Autodesk Inventor part; units mm, degrees
ref_plane "YZ Plane" through (0, 0, 0) normal (1, 0, 0) x (0, 1, 0)
ref_plane "XZ Plane" through (0, 0, 0) normal (0, 1, 0) x (-1, 0, 0)
ref_plane "XY Plane" through (0, 0, 0) normal (0, 0, 1) x (1, 0, 0)
sketch "Boceto1" plane through (0, 0, 0) normal (0, 1, 0) x (-1, 0, 0)
  line L0 (0, 0) -> (12.5, 0)
  line L1 (12.5, 0) -> (12.5, -5)
  line L2 (0, -5) -> (0, 0)
  circle A0 centre (6.25, -2.5) radius 1
  arc A1 (8.4861, -5) -> (4.0139, -5) centre (6.25, -7) ccw
  line L3 (12.5, -5) -> (8.4861, -5)
  line L4 (4.0139, -5) -> (0, -5)
  dimension "d1" = 5
  dimension "d2" = 2
  dimension "d4" = 6
extrude "Extrusión1" add sketch "Boceto1" along normal blind 5
sketch "Boceto2" plane through (0, 5, 0) normal (0, 1, 0) x (1, 0, 0)
  line L0 (0, 5) -> (-4.0139, 5)
  arc A0 (-8.4861, 5) -> (-4.0139, 5) centre (-6.25, 7) ccw
  line L1 (-8.4861, 5) -> (-12.5, 5)
  line L2 (-12.5, 5) -> (-12.5, 0)
  line L3 (-12.5, 0) -> (0, 0)
  line L4 (0, 0) -> (0, 5)
  circle A1 centre (-6.25, 2.5) radius 1
  arc A2 (-12.5, 11.25) -> (0, 11.25) centre (-6.25, 11.25) ccw
  arc A3 (0, 15.25) -> (-12.5, 15.25) centre (-6.25, 15.25) ccw
  line L5 (-12.5, 11.25) -> (-12.5, 15.25)
  line L6 (0, 11.25) -> (0, 15.25)
  line L7 (0, 23.25) -> (-12.5, 23.25)
  line L8 (-12.5, 23.25) -> (-12.5, 28.25)
  line L9 (-12.5, 28.25) -> (0, 28.25)
  line L10 (0, 28.25) -> (0, 23.25)
  circle A4 centre (-6.25, 25.75) radius 1
  circle A5 centre (-6.25, 7) radius 27
  circle A6 centre (-6.25, 7) radius 30
  dimension "d8" = 12.5
  dimension "d10" = 12.5
  dimension "d12" = 12.5
  dimension "d13" = 5
  dimension "d14" = 2
  dimension "d15" = 54
  dimension "d17" = 3
extrude "Extrusión2" add sketch "Boceto2" along normal blind 3 contours A5
extrude "Extrusión3" add sketch "Boceto2" against normal blind 5 contours L7 L8 L9 L10
extrude "Extrusión4" add sketch "Boceto2" along normal blind 6.8 contours A6
sketch "Boceto3" plane through (0, 5, 0) normal (0, 1, 0) x (1, 0, 0)
  line L0 (-4.0139, 5) -> (0, 5)
  line L1 (0, 0) -> (-12.5, 0)
  line L2 (0, 5) -> (-12.5, 5)
  line L3 (-12.5, 5) -> (-12.5, 0)
  line L4 (-12.5, 0) -> (0, 0)
  line L5 (0, 0) -> (0, 5)
  line L6 (-12.5, 28.25) -> (0, 28.25)
  line L7 (0, 23.25) -> (-12.5, 23.25)
  line L8 (0, 28.25) -> (-12.5, 28.25)
  line L9 (-12.5, 28.25) -> (-12.5, 23.25)
  line L10 (-12.5, 23.25) -> (0, 23.25)
  line L11 (0, 23.25) -> (0, 28.25)
  circle A0 centre (-6.25, 25.75) radius 1
  circle A1 centre (-6.25, 25.75) radius 1
  circle A2 centre (-6.25, 2.5) radius 1
  circle A3 centre (-6.25, 2.5) radius 1
  dimension "d24" = 12.5
  dimension "d25" = 5
  dimension "d26" = 12.5
  dimension "d27" = 5
  dimension "d28" = 2
  dimension "d29" = 2
extrude "Extrusión5" add sketch "Boceto3" along normal blind 3
sketch "Boceto4" plane through (-6.25, 5, -7) normal (0, -1, 0) x (1, 0, 0)
  circle A0 centre (0, 0) radius 27
  circle A1 centre (0, 0) radius 30
  circle A2 centre (0, 0) radius 27
  point P0 (6.25, 7)
  dimension "d32" = 60
  dimension "d33" = 54
extrude "Extrusión6" add sketch "Boceto4" along normal blind 25
sketch "Boceto5" plane through (-6.25, -20, -7) normal (0, -1, 0) x (1, 0, 0)
  circle A0 centre (0, 0) radius 27
  arc A1 (6.25, -4.25) -> (-6.25, -4.25) centre (0, -4.25) ccw
  line L0 (6.25, -8.25) -> (6.25, -4.25)
  arc A2 (-6.25, -8.25) -> (6.25, -8.25) centre (0, -8.25) ccw
  line L1 (-6.25, -4.25) -> (-6.25, -8.25)
  arc A3 (2.2361, 2) -> (-2.2361, 2) centre (0, 0) ccw
  line L2 (-2.2361, 2) -> (-6.25, 2)
  line L3 (-6.25, 2) -> (-6.25, 7)
  line L4 (-6.25, 7) -> (6.25, 7)
  line L5 (6.25, 7) -> (6.25, 2)
  line L6 (6.25, 2) -> (2.2361, 2)
  line L7 (6.25, -16.25) -> (-6.25, -16.25)
  line L8 (6.25, -21.25) -> (6.25, -16.25)
  line L9 (-6.25, -21.25) -> (6.25, -21.25)
  line L10 (-6.25, -16.25) -> (-6.25, -21.25)
  circle A4 centre (0, 0) radius 30
  circle A5 centre (0, 0) radius 27
  circle A6 centre (0, 0) radius 40
  circle A7 centre (0, 0) radius 30
  line L11 (0, 30) -> (5, 30)
  line L12 (5, 30) -> (-5, 30)
  line L13 (-5, 30) -> (-5, 26.533)
  circle A8 centre (0, 0) radius 27
  line L14 (5, 30) -> (5, 26.533)
  circle A9 centre (0, 0) radius 27
  circle A10 centre (0, 0) radius 30
  dimension "d36" = 80
  dimension "d37" = 5
  dimension "d38" = 10
extrude "Extrusión7" add sketch "Boceto5" along normal blind 3 contours A0 L14 A4 L13 | A0 L13 A4 L14 | A4 L11 L14 | L13 L12 A4 | A6
sketch "Boceto6" plane through (-6.25, -23, -7) normal (0, -1, 0) x (1, 0, 0)
  circle A0 centre (0, 0) radius 30
  circle A1 centre (0, 0) radius 40
  circle A2 centre (0, 0) radius 27
  circle A3 centre (0, 0) radius 30
  circle A4 centre (0, 0) radius 30
  circle A5 centre (0, 0) radius 40
  arc A6 (42.4961, -3.1256) -> (42.4568, 3.1566) centre (40, 0) ccw
  circle A7 centre (40, 0) radius 2.5
  circle A8 centre (0, 0) radius 40
  arc A9 (42.4961, -3.1256) -> (39.2164, -7.8789) centre (48.7365, -10.9396) ccw
  line L0 (39.8, 3.995) -> (39.8, 3.995)
  arc A10 (39.3287, 7.2975) -> (42.4568, 3.1566) centre (48.5987, 11.0482) ccw
  arc A11 (3.1545, 42.4596) -> (-3.1252, 42.4966) centre (0, 40) ccw
  circle A12 centre (0, 40) radius 2.5
  line L1 (3.995, 39.8) -> (3.995, 39.8)
  line L2 (9.1155, 38.7955) -> (7.182, 39.1748)
  arc A13 (3.1545, 42.4596) -> (9.1155, 38.7955) centre (11.0406, 48.6084) ccw
  line L3 (-3.995, 39.8) -> (-3.995, 39.8)
  line L4 (-9.2166, 38.8873) -> (-9.7422, 38.7955)
  arc A14 (-9.2166, 38.8873) -> (-3.1252, 42.4966) centre (-10.9383, 48.738) ccw
  arc A15 (-3.2297, -42.3598) -> (3.1372, -42.4816) centre (0, -40) ccw
  circle A16 centre (0, -40) radius 2.5
  arc A17 (-42.4596, 3.1545) -> (-42.4753, -3.1421) centre (-40, 0) ccw
  circle A18 centre (-40, 0) radius 2.5
  line L5 (-8.8392, -38.5679) -> (-8.6091, -38.6265)
  arc A19 (7.6163, -39.2682) -> (3.1372, -42.4816) centre (10.9801, -48.6855) ccw
  arc A20 (-3.2297, -42.3598) -> (-6.5544, -39.4593) centre (-11.3041, -48.2594) ccw
  arc A21 (-42.4596, 3.1545) -> (-39.3229, 7.3286) centre (-48.6084, 11.0406) ccw
  arc A22 (-39.2858, -7.5248) -> (-42.4753, -3.1421) centre (-48.6635, -10.9974) ccw
  point P0 (6.25, 7)
  point P1 (39.8, -3.995)
  point P2 (3.995, -39.8)
  point P3 (-3.995, -39.8)
  point P4 (-39.8, -3.995)
  point P5 (-39.8, 3.995)
  point P6 (-39.2858, -7.5248)
  point P7 (-39.9219, -2.4988)
  point P8 (-39.9219, 2.4988)
  point P9 (-39.3229, 7.3286)
  point P10 (-7.8886, 39.2144)
  point P11 (-2.4988, 39.9219)
  point P12 (2.4988, 39.9219)
  point P13 (7.3286, 39.3229)
  point P14 (2.4988, -39.9219)
  point P15 (-2.4988, -39.9219)
  point P16 (-6.5544, -39.4593)
  point P17 (39.3287, 7.2975)
  point P18 (39.9219, 2.4988)
  point P19 (39.9219, -2.4988)
  dimension "d41" = 8
  dimension "d42" = 5
  dimension "d43" = 10
  dimension "d44" = 10
  dimension "d45" = 8
  dimension "d46" = 5
  dimension "d47" = 10
  dimension "d48" = 10
  dimension "d49" = 8
  dimension "d50" = 5
  dimension "d51" = 8
  dimension "d52" = 5
  dimension "d53" = 10
  dimension "d54" = 10
extrude "Extrusión8" add sketch "Boceto6" against normal blind 3 contours A1 A18 A22 A17 A21 | A14 A11 A13 A1 A12 | A1 A16 A19 A15 A20 | A10 A6 A9 A1 A7
extrude "Extrusión9" cut sketch "Boceto6" against normal blind 3 contours A18 A1 | A1 A12 | A16 A1 | A1 A7 picked at (-39.1609, 0) picked at (-0.0985, 39.1667) picked at (-0.0985, -39.1667) picked at (39.2158, -0.5677)
sketch "Boceto7" plane through (0, 0, 0) normal (0, 0, 1) x (1, 0, 0)
  line L0 (-36.25, -20) -> (23.75, -20)
  line L1 (23.75, 11.8) -> (-36.25, 11.8)
  line L2 (-3.0955, -23) -> (-9.3752, -23)
  line L3 (-3.0955, -23) -> (-3.0955, -20)
  line L4 (-9.3752, -20) -> (-3.0955, -20)
  line L5 (-9.3752, -23) -> (-9.3752, -20)
  line L6 (1.0786, -23) -> (-3.0955, -23)
  line L7 (1.0786, -20) -> (1.0786, -23)
  line L8 (-3.0955, -20) -> (1.0786, -20)
  line L9 (-3.0955, -23) -> (-3.0955, -20)
  line L10 (-12.8044, -20) -> (-12.8044, -23)
  line L11 (-9.3752, -23) -> (-14.1386, -23)
  line L12 (-9.3752, -23) -> (-9.3752, -20)
  line L13 (-14.1386, -20) -> (-9.3752, -20)
  line L14 (-14.1386, -23) -> (-14.1386, -20)
  line L15 (-3.75, -20) -> (-3.75, -23)
  line L16 (-3.75, -21.5) -> (-8.75, -21.5)
  line L17 (-6.25, -22.5562) -> (-1.25, -22.5562)
  line L18 (-1.25, -22.5562) -> (-11.25, -22.5562)
  line L19 (-11.25, -22.5562) -> (-11.25, -20)
  line L20 (-11.25, -20) -> (-1.25, -20)
  line L21 (-1.25, -20) -> (-1.25, -15)
  line L22 (-1.25, -15) -> (-11.25, -15)
  line L23 (-11.25, -15) -> (-11.25, -20)
  point P0 (0, 0)
  dimension "d59" = 5
  dimension "d60" = 5
  dimension "d61" = 10
  dimension "d62" = 10
  dimension "d63" = 5
extrude "Extrusión10" cut sketch "Boceto7" along normal blind 30 contours L23 L22 L21 L0
properties part number "Pieza1parte3"
Work out the finished part from the listing and answer in its coordinate system (mm). A direction names the side the tool comes from. Give positions to 0.01 mm unless a question says otherwise; leave off trailing zeros. Order: outer loops, then holes, each group sorted by start corner. A loop starts at its lowest first (then second) coordinate and runs counter-clockwise, first axis right, second up.
1. Straight lines are drawn through the part: L1, parallel to Z at x = -6.25, y = 5.25; L2, parallel to Z at x = -6, y = -21; L3, parallel to Z at x = -6, y = -2. For each, find the intervals that lie inside material, in ascending order.
Result sheet:
L1: z = -37 to -26.75, -24.75 to -21.5, -5 to -3.5, -1.5 to 23
L2: z = -50.99 to -49.49, -44.51 to -34, 20 to 30.51, 35.49 to 36.99
L3: z = -37 to -34, 20 to 23
2. Section B-B, the plane z = -13 is taken. Determine the outline of the cut face in (x, y).
Result sheet:
outline: (-46.25, -23) - (-32.57, -23) - (-32.57, 5) - (-12.5, 5) - (-12.5, 8) - (-32.57, 8) - (-32.57, 11.8) - (-35.64, 11.8) - (-35.64, -20) - (-46.25, -20) - close; (0, 5) - (20.07, 5) - (20.07, -23) - (33.79, -23) - (33.79, -20) - (23.14, -20) - (23.14, 11.8) - (20.07, 11.8) - (20.07, 8) - (0, 8) - close
3. The mould has two halves that part along Z. Classify faces 1 (the flat face through (-26, -20, -30)), 2 (the cylindrical face through (-1.2, -21.5, 33.6)), 3 (the flat face through (-7, 8, -1)): released by +Z, released by -Z, zero draft, split by the parting line, or undercut.
Result sheet:
face 1: zero draft
face 2: released by +Z
face 3: undercut
4. Section C-C, the plane x = 16.5 is taken. Determine the outline of the cut face in (y, z), and give its area (3 significant figures).
Result sheet:
outline: (-23, -39.9) - (-20, -39.9) - (-20, -26.56) - (11.8, -26.56) - (11.8, -21.54) - (8, -21.54) - (8, 7.54) - (11.8, 7.54) - (11.8, 12.56) - (-20, 12.56) - (-20, 25.9) - (-23, 25.9) - (-23, 7.54) - (5, 7.54) - (5, -21.54) - (-23, -21.54) - close
area: 516 mm2
5. Section D-D, the plane z = 15 is taken. Determine the outline of the cut face in (x, y).
Result sheet:
outline: (-39.66, -23) - (-21.9, -23) - (-21.9, 5) - (9.4, 5) - (9.4, -23) - (27.16, -23) - (27.16, -20) - (14.15, -20) - (14.15, 11.8) - (9.4, 11.8) - (9.4, 8) - (-21.9, 8) - (-21.9, 11.8) - (-26.65, 11.8) - (-26.65, -20) - (-39.66, -20) - close
6. Each of these flat-tipped pins is pushed along its axis until it touches: P1, Ø1.5, axis at x = -6, y = 2, coming from the +Z side; P2, Ø1.5, axis at y = -18.5, z = 20.5, coming from the +X side; P3, Ø1, axis at x = -18.5, y = -4.5, coming from the -Z side; P4, Ø1.2, axis at x = -6.25, z = -2.5, coming from the +Y side. Where does it stop, or does it pass through?
Result sheet:
P1: stops at z = 23
P2: stops at x = 7.33
P3: stops at z = -34.6
P4: passes through
7. Section A-A, the plane y = 2 is taken. Determine the outline of the cut face in (x, z), and give its area (3 significant figures).
Result sheet:
outline: circle Ø60 at (-6.25, -7); (-12.5, -28.25) - (0, -28.25) - (0, -23.25) - (-12.5, -23.25) - close; (-12.5, -5) - (-8.49, -5) arc R3 cw to (-4.01, -5) - (0, -5) - (0, 0) - (-12.5, 0) - close; hole circle Ø54 at (-6.25, -7); hole circle Ø2 at (-6.25, -25.75); hole circle Ø2 at (-6.25, -2.5)
area: 653 mm2
8. For faces 4 (the cylindrical face through (-28, -9, 9)), 5 (the flat face through (-12.5, 6, -13)), 6 (the cylindrical face through (-50.25, -21.52, -6.94)), 7 (the flat face through (-11.25, -17, 21)), determine the directions among +Z, -Z, +X, -X, +Y, -Y from which every point of the face is accessible in a straight line to the end or side of a thin tool.
Result sheet:
face 4: -Y
face 5: +Y, -Y
face 6: -X, +Y, -Y
face 7: +Z
